```python
from build123d import *

# Parameters (mm, degrees)
F0_W          = 120
F0_H          = 80
F0_W_2        = 108
F0_H_2        = 68
F1_DEPTH      = 25
F3_DEPTH      = 80.001
F5_DEPTH      = 60.001
F5_DEPTH_BACK = 60.001
F6_W          = 120
F6_H          = 80
F6_W_2        = 114
F6_H_2        = 74
F7_DEPTH      = 5
F8_R          = 5
F9_R          = 2
F10_R         = 0.5
F11_R         = 2


with BuildPart() as f1:
    # F0 (on Top) → F1 (new body)
    with BuildSketch(Plane.XY):
        Rectangle(F0_W, F0_H)
        Rectangle(F0_W_2, F0_H_2, mode=Mode.SUBTRACT)
    extrude(amount=F1_DEPTH)

    # F2 (on face) → F3 (cut, through all)
    with BuildSketch(Plane.XZ.offset(40)):
        Polygon((-57.8127834119, 0), (-60, 25), (-75, 25), (-75, -19.6831412613), (75, -19.6831412613), (75, 25), (60, 25), (57.8127834119, 0), align=None)
    extrude(amount=-F3_DEPTH, mode=Mode.SUBTRACT)

    # F4 (on Right) → F5 (cut, two sides)
    with BuildSketch(Plane.YZ) as f5_sk:
        Polygon((55, 25), (40, 25), (37.8127834119, 0), (-37.8127834119, 0), (-40, 25), (-55, 25), (-55, -15), (55, -15), align=None)
    extrude(amount=-F5_DEPTH, mode=Mode.SUBTRACT)
    extrude(f5_sk.sketch, amount=F5_DEPTH_BACK, mode=Mode.SUBTRACT)

    # F6 (on face) → F7 (cut)
    with BuildSketch(Plane.XY.offset(25)):
        Rectangle(F6_W, F6_H)
        Rectangle(F6_W_2, F6_H_2, mode=Mode.SUBTRACT)
    extrude(amount=-F7_DEPTH, mode=Mode.SUBTRACT)

    # F8
    f8_edges = [f1.edges().sort_by_distance(p)[0] for p in [
        (-57, -37, 22.5),
        (-57, 37, 22.5),
        (57, -37, 22.5),
        (57, 37, 22.5),
    ]]
    fillet(f8_edges, radius=F8_R)

    # F9
    f9_edges = [f1.edges().sort_by_distance(p)[0] for p in [
        (-58.68767, -38.68767, 10),
        (-58.68767, 38.68767, 10),
        (58.68767, -38.68767, 10),
        (58.68767, 38.68767, 10),
    ]]
    fillet(f9_edges, radius=F9_R)

    # F10
    f10_edges = [f1.edges().sort_by_distance(p)[0] for p in [
        (0, -39.562557, 20),
    ]]
    fillet(f10_edges, radius=F10_R)

    # F11
    f11_edges = [f1.edges().sort_by_distance(p)[0] for p in [
        (-54, 34, 12.5),
        (-54, -34, 12.5),
        (54, -34, 12.5),
        (54, 34, 12.5),
    ]]
    fillet(f11_edges, radius=F11_R)


solid = f1.part
```
Geometry check sheet. Reference: the model listing, model coordinates, mm. A direction names the side the tool comes from. Coordinates: 2 decimals unless noted, no trailing zeros. Order: outer loops, then holes, each group sorted by start corner. A loop starts at its lowest first (then second) coordinate and runs counter-clockwise, first axis right, second up. Notation, with made-up numbers: (47, 41) - (87, 41) arc R14 ccw to (87, 68) - close; hole circle Ø3 at (77.25, -6.5). An arc over 180 degrees is marked (long way). Answer in a Markdown table with one row per item. Add a question column.
1. Access from +Z, -Z, +X, -X, +Y, -Y to the whole of each face (thin tool, end or side, straight path). Record for faces 1 (the face through (-56, 35, 22)), 2 (the face through (56, -35, 22)), 3 (the face through (-1, -34, 12)).
2. Section check B-B (y = 3). Enter the section's corners in (x, z) (3 decimals), plus the area to 3 significant figures.
3. Draft check along X on faces 4 (the face through (58.105, -38.074, 9.82)), 5 (the face through (-58.65, -0.53, 9.59)), 6 (the face through (-1, 34, 12)), 7 (the face through (-1, 37, 23)). Enter one of: +X half, -X half, draft (parallel to the pull), parting line (faces both ways), or undercut.
4. Gauge pin test, flat ends, axial feed: pin 1 Ø5 at (y, z) = (-14.5, 14) entering from +X; pin 2 Ø1.5 at (y, z) = (0, 22) entering from +X; pin 3 Ø2 at (y, z) = (21.5, 15) entering from -X. Record the tip position at first contact, or that the pin passes through.
5. Material ranges on L1, parallel to X at y = -31, z = 13.5; L2, parallel to X at y = -16, z = 21.75; L3, parallel to Y at x = -4, z = 23.5, recorded low to high. Write a range as [from, to].
6. Section check A-A (x = -37). Enter the section's corners in (y, z) (3 decimals), plus the area to 3 significant figures.
Data:
| question | item | result |
|---|---|---|
| 1 | face 1 | +Z, -X, +Y |
| 1 | face 2 | +Z, +X, -Y |
| 1 | face 3 | +Z, -Z |
| 2 | outline | (-59.515, 19.456) - (-57.813, 0) - (-54, 0) - (-54, 25) - (-57, 25) - (-57, 20) - (-59.017, 20) arc R0.5 ccw to start; (54, 0) - (57.813, 0) - (59.515, 19.456) arc R0.5 ccw to (59.017, 20) - (57, 20) - (57, 25) - (54, 25) - close |
| 2 | area | 217 mm² |
| 3 | face 4 | +X half |
| 3 | face 5 | -X half |
| 3 | face 6 | undercut |
| 3 | face 7 | draft |
| 4 | pin 1 | stops at x = 59.26 |
| 4 | pin 2 | stops at x = 57 |
| 4 | pin 3 | stops at x = -59.21 |
| 5 | L1 | x = [-58.99, -54], [54, 58.99] |
| 5 | L2 | x = [-57, -54], [54, 57] |
| 5 | L3 | y = [-37, -34], [34, 37] |
| 6 | outline | (-39.515, 19.456) - (-37.813, 0) - (-34, 0) - (-34, 25) - (-37, 25) - (-37, 20) - (-39.017, 20) arc R0.5 ccw to start; (34, 0) - (37.813, 0) - (39.515, 19.456) arc R0.5 ccw to (39.017, 20) - (37, 20) - (37, 25) - (34, 25) - close |
| 6 | area | 217 mm² |
